from build123d import *

# Parameters (mm, degrees)
EXTRUDE_1_DEPTH     = 10
CUT_EXTRUDE_1_DEPTH = 54
CUT_EXTRUDE_2_DEPTH = 54
EXTRUDE_START       = 10
EXTRUDE_2_DEPTH     = 10
EXTRUDE_START_2     = -10
EXTRUDE_3_DEPTH     = 10
EXTRUDE_4_DEPTH     = 10
CUT_EXTRUDE_3_DEPTH = 10
SKETCH_9_R          = 1.3
CUT_EXTRUDE_4_DEPTH = 8
CHAMFER_1_SIZE      = 3
CHAMFER_2_SIZE      = 3
CHAMFER_3_SIZE      = 1
CHAMFER_4_SIZE      = 0.5
FILLET_1_R          = 0.5


with BuildPart() as part:
    # 草图1 → 凸台-拉伸1 (new body)
    with BuildSketch(Plane.XY):
        with BuildLine():
            Line((-10, 0), (-19, 0))
            Line((-19, 0), (-19, -6))
            Line((-19, -6), (-13.747727085, -6))
            ThreePointArc((-13.747727085, -6), (-11.184043696, -9.995857472), (-7.5, -12.990381057))
            Line((-7.5, -12.990381057), (-7.5, -29))
            Line((-7.5, -29), (7.5, -29))
            Line((7.5, -29), (7.5, -12.990381057))
            ThreePointArc((7.5, -12.990381057), (11.184043696, -9.995857472), (13.747727085, -6))
            Line((13.747727085, -6), (19, -6))
            Line((19, -6), (19, 0))
            Line((19, 0), (10, 0))
            ThreePointArc((10, 0), (0, -10), (-10, 0))
        make_face()
    extrude(amount=EXTRUDE_1_DEPTH)

    # 草图3 → 切除-拉伸1 (cut)
    with BuildSketch(Plane(origin=(7.5, 0, 0), x_dir=(0, 0, -1), z_dir=(1, 0, 0))):
        with BuildLine():
            Line((-3.86862915, -23.86862915), (-2.7372583, -25))
            Line((-2.7372583, -25), (-3.86862915, -26.13137085))
            ThreePointArc((-3.86862915, -26.13137085), (-6.6, -25), (-3.86862915, -23.86862915))
        make_face()
    extrude(amount=-CUT_EXTRUDE_1_DEPTH, mode=Mode.SUBTRACT)

    # 草图4 → 切除-拉伸2 (cut)
    with BuildSketch(Plane(origin=(0, 0, 0), x_dir=(1, 0, 0), z_dir=(0, 1, 0))):
        with BuildLine():
            Line((-15, -3.161522369), (-15.919238816, -4.080761184))
            ThreePointArc((-15.919238816, -4.080761184), (-15, -6.3), (-14.080761184, -4.080761184))
            Line((-14.080761184, -4.080761184), (-15, -3.161522369))
        make_face()
        with BuildLine():
            Line((15, -3.161522369), (14.080761184, -4.080761184))
            ThreePointArc((14.080761184, -4.080761184), (15, -6.3), (15.919238816, -4.080761184))
            Line((15.919238816, -4.080761184), (15, -3.161522369))
        make_face()
    extrude(amount=-CUT_EXTRUDE_2_DEPTH, mode=Mode.SUBTRACT)

    # 草图5 → 凸台-拉伸2 (add)
    with BuildSketch(Plane(origin=(0, 0, 0), x_dir=(-1, 0, 0), z_dir=(0, 0, -1)).offset(EXTRUDE_START)):
        with BuildLine():
            Line((-15, 0), (-10, 0))
            ThreePointArc((-10, 0), (0, -10), (10, 0))
            Line((10, 0), (15, 0))
            ThreePointArc((15, 0), (0, -15), (-15, 0))
        make_face()
    extrude(amount=-EXTRUDE_2_DEPTH)

    # 草图6 → 凸台-拉伸3 (add)
    with BuildSketch(Plane.XY.offset(10).offset(EXTRUDE_START_2)):
        with BuildLine():
            Line((-13.747727085, -6), (-16.970562748, -6))
            ThreePointArc((-16.970562748, -6), (0, -18), (16.970562748, -6))
            Line((16.970562748, -6), (13.747727085, -6))
            ThreePointArc((13.747727085, -6), (0, -15), (-13.747727085, -6))
        make_face()
    extrude(amount=EXTRUDE_3_DEPTH)

    # 草图7 → 凸台-拉伸4 (add)
    with BuildSketch(Plane(origin=(0, 0, 0), x_dir=(-1, 0, 0), z_dir=(0, 0, -1)).offset(EXTRUDE_START)):
        with BuildLine():
            Line((-15, 0), (-19, 0))
            Line((-19, 0), (-19, -6))
            Line((-19, -6), (-16.970562748, -6))
            Line((-16.970562748, -6), (-13.747727085, -6))
            ThreePointArc((-13.747727085, -6), (-14.683594694, -3.064644655), (-15, 0))
        make_face()
        with BuildLine():
            ThreePointArc((15, 0), (14.683594694, -3.064644655), (13.747727085, -6))
            Line((13.747727085, -6), (16.970562748, -6))
            Line((16.970562748, -6), (19, -6))
            Line((19, -6), (19, 0))
            Line((19, 0), (15, 0))
        make_face()
    extrude(amount=-EXTRUDE_4_DEPTH)

    # 草图8 → 切除-拉伸3 (cut)
    with BuildSketch(Plane(origin=(0, 0, 0), x_dir=(1, 0, 0), z_dir=(0, 1, 0))):
        with BuildLine():
            Line((-15, 6.838477631), (-15.919238816, 5.919238816))
            ThreePointArc((-15.919238816, 5.919238816), (-15, 3.7), (-14.080761184, 5.919238816))
            Line((-14.080761184, 5.919238816), (-15, 6.838477631))
        make_face()
        with BuildLine():
            Line((15, 6.838477631), (14.080761184, 5.919238816))
            ThreePointArc((14.080761184, 5.919238816), (15, 3.7), (15.919238816, 5.919238816))
            Line((15.919238816, 5.919238816), (15, 6.838477631))
        make_face()
    extrude(amount=-CUT_EXTRUDE_3_DEPTH, mode=Mode.SUBTRACT)

    # 草图9 → 切除-拉伸4 (cut)
    with BuildSketch(Plane.XY.offset(10)):
        with Locations((-9.899494937, -9.899494937)):
            Circle(SKETCH_9_R)
        with Locations(Location((9.899494937, -9.899494937, 0), (0, 0, 180))):
            Circle(SKETCH_9_R)
    extrude(amount=-CUT_EXTRUDE_4_DEPTH, mode=Mode.SUBTRACT)

    # 倒角1
    chamfer_1_edges = [part.edges().sort_by_distance(p)[0] for p in [
        (0, -15, 0),
    ]]
    chamfer(chamfer_1_edges, length=CHAMFER_1_SIZE - 0.0001)  # a hair under: the kernel refuses the full size

    # 倒角2
    chamfer_2_edges = [part.edges().sort_by_distance(p)[0] for p in [
        (0, -29, 0),
        (0, -29, 10),
    ]]
    chamfer(chamfer_2_edges, length=CHAMFER_2_SIZE)

    # 倒角3
    chamfer_3_edges = [part.edges().sort_by_distance(p)[0] for p in [
        (-19, -3, 10),
        (19, -3, -10),
        (-19, -3, -10),
        (19, -3, 10),
    ]]
    chamfer(chamfer_3_edges, length=CHAMFER_3_SIZE)

    # 倒角4
    chamfer_4_edges = [part.edges().sort_by_distance(p)[0] for p in [
        (0, -15, -10),
        (-11.199494937, -9.899494937, 2),
        (-11.199494937, -9.899494937, 10),
        (11.199494937, -9.899494937, 2),
        (11.199494937, -9.899494937, 10),
        (15.873863542, -6, -10),
        (-15.873863542, -6, -10),
        (-14, 0, -10),
        (-7.5, -25, 6.6),
        (-7.5, -24.434314575, 3.302943725),
        (-7.5, -25.565685425, 3.302943725),
        (7.5, -25, 6.6),
        (7.5, -25.565685425, 3.302943725),
        (7.5, -24.434314575, 3.302943725),
        (0, -10, 10),
        (0, -10, -10),
        (14, 0, -10),
    ]]
    chamfer(chamfer_4_edges, length=CHAMFER_4_SIZE)

    # 圆角1
    fillet_1_edges = [part.edges().sort_by_distance(p)[0] for p in [
        (10, 0, 0),
        (-10, 0, 0),
    ]]
    fillet(fillet_1_edges, radius=FILLET_1_R)


solid = part.part
Verification items for the finished model (mm, model axes). A direction names the side the tool comes from. Coordinates: 2 decimals unless noted, no trailing zeros. Order: outer loops, then holes, each group sorted by start corner. A loop starts at its lowest first (then second) coordinate and runs counter-clockwise, first axis right, second up. Notation, with made-up numbers: M 71.25,87 L 81.25,87 A16 cw 81.25,96 Z; hole C -18.5,74 d11. An arc over 180 degrees is marked long. One line per item, written item: value. Start each with the question number.
Item 1: Depth check by flat-ended pin: P1, Ø1, axis at x = 0, y = -17.5, coming from the -Z side; P2, Ø5, axis at y = -23, z = 3.5, coming from the -X side; P3, Ø2, axis at x = 15, z = 5, coming from the -Y side; P4, Ø1, axis at x = 9, y = -16.5, coming from the +Z side. Enter the tip coordinate at first touch or a pass-through.
Item 2: Thickness scan on probe 1 along X at (y, z) = (-4.75, 5); probe 2 along Y at (x, z) = (3, 5); probe 3 along Y at (x, z) = (-7, 4.75). Record the ranges inside material, lowest first.
Item 3: Access from +Z, -Z, +X, -X, +Y, -Y to the whole of each face (thin tool, end or side, straight path). Record for faces 4 (the flat face through (-7.247, -24.282, 3.106)), 5 (the flat face through (-17, -6, -2)), 6 (the flat face through (15.47, -2.96, 3.63)), 7 (the flat face through (15.47, -2.96, -6.37)).
Item 4: Sectioned sample at C-C on y = -2.5. Give the number of separate pieces and of enclosed holes in the cut face, then the cut area to 3 significant figures.
Item 5: Sectioned sample at A-A on x = 0. Record the cut outline in (y, z).
Item 6: Mould release check, pull along Z, two halves, no side actions. Record for faces 1 (the flat face through (10, -10, 2)), 2 (the flat face through (-7.5, -21, 5)), 3 (the flat face through (0.1, -24.43, 3.31)): pulls with the +Z half, pulls with the -Z half, needs draft (parallel to the pull), parting line crosses it, or undercut.
Item 7: Sectioned sample at B-B on z = -1.75. Record the cut outline in (x, y).
Calculated:
1. P1: z = -1
1. P2: x = -7.5
1. P3: y = -11.31
1. P4: through
2. probe 1: -19 to -16.3, -13.7 to -8.8, 8.8 to 13.7, 16.3 to 19
2. probe 2: -29 to -26.6, -23.4 to -9.54
2. probe 3: -29 to -26.58, -23.42 to -7.14
3. face 4: -X
3. face 5: -Z, -X, -Y
3. face 6: +Y
3. face 7: +Y, -Y
4. separate pieces: 2
4. enclosed holes: 4
4. area: 347 mm^2
5. outline: M -29,3 L -26,0 L -18,0 L -15,-3 L -15,-9.5 L -14.5,-10 L -10.5,-10 L -10,-9.5 L -10,9.5 L -10.5,10 L -26,10 L -29,7 Z; hole M -26.13,3.87 L -25,2.74 L -23.87,3.87 A1.6 ccw long Z
6. face 1: pulls with the +Z half
6. face 2: needs draft
6. face 3: undercut
7. outline: M -19,-6 L -15.1,-6 A16.25 ccw 15.1,-6 L 19,-6 L 19,0 L 10.49,0 A0.5 ccw 9.99,-0.48 A10 cw -9.99,-0.48 A0.5 ccw -10.49,0 L -19,0 Z
